Verification items for this drawing (mm, ordinates from the low corner). Coordinates: 2 decimals unless noted, no trailing zeros. Loops run counter-clockwise (first coordinate to the right, second up) from the corner with the lowest first, then second, coordinate; pieces in that order, holes last. Notation, with made-up numbers: M -4.75,7 L 54.25,7 A22 cw 54.25,46 Z; hole C 32.25,-3.5 d9. An arc over 180 degrees is marked long. Use CSV: the item, a comma, the result in double quotes.
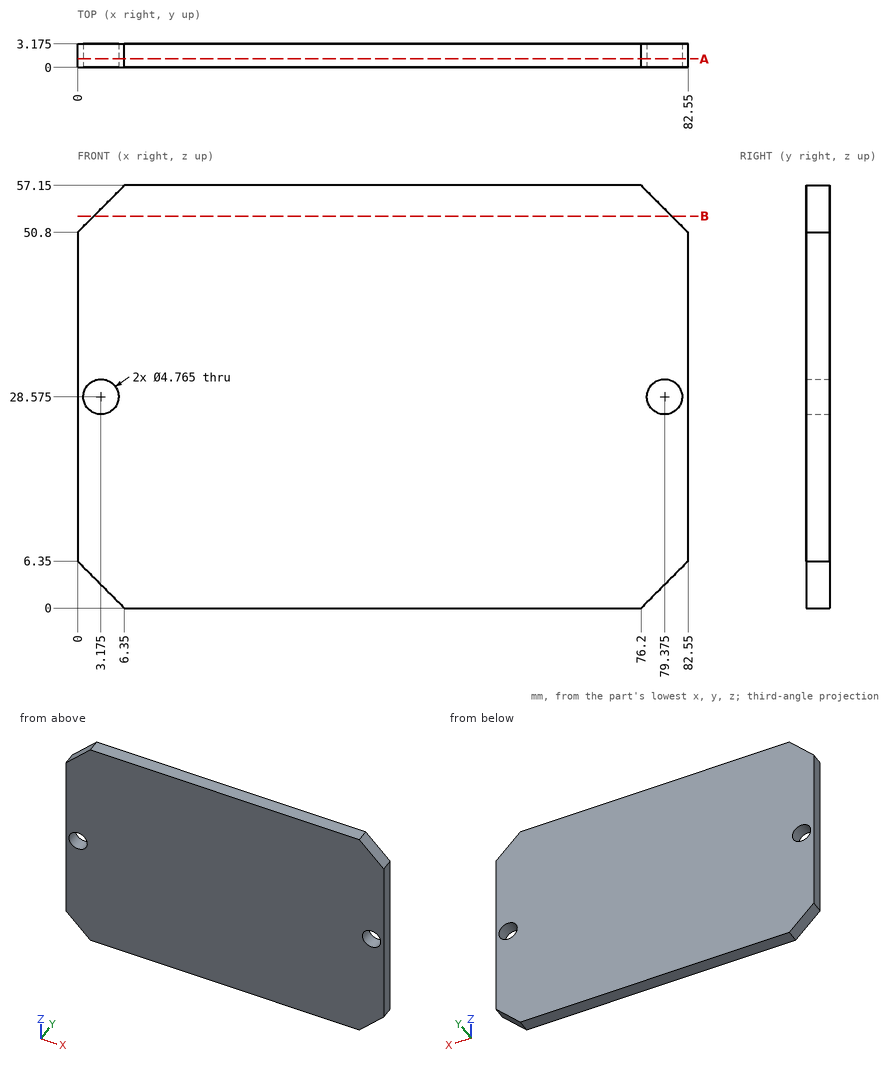
1. Thickness scan on line 1 (X direction, y = 1.9, z = 30.5); line 2 (X direction, y = 1.8, z = 27); line 3 (Z direction, x = 77.5, y = 0.45) (3 decimals). Record the ranges inside material, lowest first. Write a range as [from, to].
The answers:
line 1,"[0, 1.77], [4.58, 77.97], [80.78, 82.55]"
line 2,"[0, 1.39], [4.96, 77.59], [81.16, 82.55]"
line 3,"[1.3, 27.105], [30.045, 55.85]"
2. Gauge pin test, flat ends, axial feed: P1, Ø3, axis at x = 79.375, z = 28.575, coming from the +Y side; P2, Ø6, axis at x = 3.175, z = 28.575, coming from the -Y side. Record the tip position at first contact, or that the pin passes through.
The answers:
P1,"through"
P2,"y = 0"
3. Section check A-A, the plane y = 1.15. Count the separate pieces of the cut face and the enclosed holes in it, plus the area to 3 significant figures.
The answers:
separate pieces,"1"
enclosed holes,"2"
area,"4,600 mm^2"
4. Section check B-B, the plane z = 53. Record the cut outline in (x, y) (3 decimals), plus the area to 3 significant figures.
The answers:
outline,"M 2.2,0 L 80.35,0 L 80.35,3.175 L 2.2,3.175 Z"
area,"248 mm^2"
